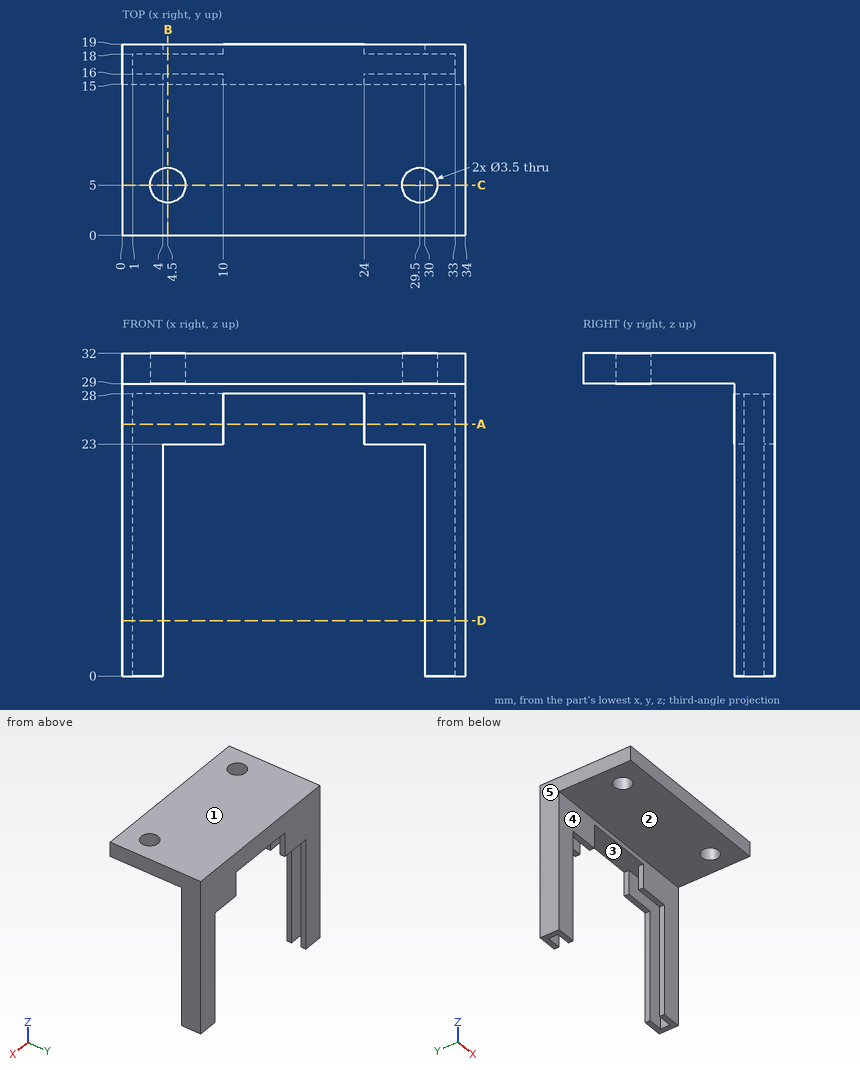
Could you check a few things on this drawing? It's one solid part, dimensions in mm from its lowest x, y, z. A direction names the side the tool comes from. Round coordinates to 2 decimals unless told otherwise and drop trailing zeros. Order: outer loops, then holes, each group sorted by start corner. A loop starts at its lowest first (then second) coordinate and runs counter-clockwise, first axis right, second up. Notation, with made-up numbers: M -17.5,2.25 L 17.5,2.25 A20 ccw 17.5,8.25 Z; hole C 46,-0.5 d10. An arc over 180 degrees is marked long. One line per question, with ' | ' between items. Start each with the question number.
(1) Suppose I cut it at A-A on z = 25. List the corners of the cut face in (x, y) for me, then the cut area to 3 significant figures.
(2) Suppose I cut it at B-B on x = 4.5. List the corners of the cut face in (y, z) for me.
(3) For P1, Ø0.8, axis at x = 7.5, y = 18.5, coming from the -Z side; P2, Ø4, axis at x = 29.5, y = 5, coming from the -Z side; P3, Ø2.5, axis at x = 3.5, z = 19.5, coming from the -Y side, each with a flat end and sliding along its axis, tell me the tip position at first contact or that it passes through.
(4) Please list where these lines run through material, in increasing order: line 1 along X through (y, z) = (5, 31.1); line 2 along X through (y, z) = (16.25, 1); line 3 along Y through (x, z) = (32, 27).
(5) Suppose I cut it at D-D on z = 5.5. List the corners of the cut face in (x, y) for me, then the cut area to 3 significant figures.
(6) Suppose I cut it at C-C on y = 5. List the corners of the cut face in (x, z) for me.
(7) Thinking about a two-plate mould opening in Y: for the marked faces 3, 4 and 5, which applies, +Y half, -Y half, draft (parallel to the pull), parting line (faces both ways), or undercut?
(8) For the marked faces 1 and 2, which set-ups out of +Z, -Z, +X, -X, +Y, -Y let a thin tool reach every point of the face, with its end or its side?
Geometry results:
1) outline: M 0,15 L 10,15 L 10,16 L 1,16 L 1,18 L 10,18 L 10,19 L 0,19 Z; M 24,15 L 34,15 L 34,19 L 24,19 L 24,18 L 33,18 L 33,16 L 24,16 Z | area: 44.0 mm²
2) outline: M 0,29 L 3.25,29 L 3.25,32 L 0,32 Z; M 6.75,29 L 15,29 L 15,23 L 16,23 L 16,28 L 18,28 L 18,23 L 19,23 L 19,32 L 6.75,32 Z
3) P1: z = 23 | P2: z = 29 | P3: y = 15
4) line 1: 0 to 2.75, 6.25 to 27.75, 31.25 to 34 | line 2: 0 to 1, 33 to 34 | line 3: 15 to 16, 18 to 19
5) outline: M 0,15 L 4,15 L 4,16 L 1,16 L 1,18 L 4,18 L 4,19 L 0,19 Z; M 30,15 L 34,15 L 34,19 L 30,19 L 30,18 L 33,18 L 33,16 L 30,16 Z | area: 20.0 mm²
6) outline: M 0,29 L 2.75,29 L 2.75,32 L 0,32 Z; M 6.25,29 L 27.75,29 L 27.75,32 L 6.25,32 Z; M 31.25,29 L 34,29 L 34,32 L 31.25,32 Z
7) face 3: undercut | face 4: -Y half | face 5: draft
8) face 1: +Z, +X, -X, +Y, -Y | face 2: -Z, +X, -X, -Y
